Input: part model. Units: mm. Frame: model coordinates. A direction names the side the tool comes from. Coordinates: 2 decimals unless noted, no trailing zeros. Write each loop counter-clockwise with the first axis right and the second up, starting at its lowest first coordinate (ties: lowest second). Pieces come first, ordered by that corner, then holes.
from build123d import *

# Parameters (mm, degrees)
SKETCH1_W           = 81
SKETCH1_H           = 29
BOSS_EXTRUDE1_DEPTH = 3
CUT_EXTRUDE2_DEPTH  = 81
CUT_EXTRUDE3_DEPTH  = 81
SKETCH6_W           = 1.85
SKETCH6_H           = 1.55
CUT_EXTRUDE5_DEPTH  = 0.6
FILLET6_R           = 0.4
CHAMFER2_SIZE       = 0.2
SKETCH7_W           = 1.85
SKETCH7_H           = 1.55
CUT_EXTRUDE6_DEPTH  = 0.6
FILLET7_R           = 0.4
CHAMFER3_SIZE       = 0.2
SKETCH11_W          = 81
SKETCH11_H          = 26.1
CUT_EXTRUDE7_DEPTH  = 0.2
FILLET8_R           = 0.4
BOSS_EXTRUDE2_DEPTH = 3
FILLET9_R           = 1
FILLET10_R          = 0.5


with BuildPart() as part:
    # Sketch1 → Boss-Extrude1 (new body)
    with BuildSketch(Plane(origin=(0, 0, 0), x_dir=(1, 0, 0), z_dir=(0, 1, 0))):
        with Locations((40.5, 14.5)):
            Rectangle(SKETCH1_W, SKETCH1_H)
    extrude(amount=BOSS_EXTRUDE1_DEPTH)

    # Sketch2 → Cut-Extrude2 (cut)
    with BuildSketch(Plane(origin=(81, 0, 0), x_dir=(0, 0, -1), z_dir=(1, 0, 0))):
        Polygon((0, 3), (3, 3), (3, 1.75), (1.25, 1.75), (1.25, 0), (0, 0), align=None)
        Polygon((29, 0), (27.75, 0), (27.75, 1.75), (26, 1.75), (26, 3), (29, 3), align=None)
    extrude(amount=-CUT_EXTRUDE2_DEPTH, mode=Mode.SUBTRACT)

    # Sketch4 → Cut-Extrude3 (cut)
    with BuildSketch(Plane(origin=(81, 0, 0), x_dir=(0, 0, -1), z_dir=(1, 0, 0))):
        Polygon((27.75, 0), (27.55, 0), (27.55, 1.55), (25.8, 1.55), (25.8, 3), (26, 3), (26, 1.75), (27.75, 1.75), align=None)
        Polygon((3.2, 3), (3, 3), (3, 1.75), (1.25, 1.75), (1.25, 0), (1.45, 0), (1.45, 1.55), (3.2, 1.55), align=None)
    extrude(amount=-CUT_EXTRUDE3_DEPTH, mode=Mode.SUBTRACT)

    # Sketch6 → Cut-Extrude5 (cut)
    with BuildSketch(Plane.XY.offset(-1.45)):
        with Locations((3, 0.775)):
            Rectangle(SKETCH6_W, SKETCH6_H)
    extrude(amount=-CUT_EXTRUDE5_DEPTH, mode=Mode.SUBTRACT)

    # Fillet6
    fillet6_edges = [part.edges().sort_by_distance(p)[0] for p in [
        (2.075, 0.775, -1.45),
    ]]
    fillet(fillet6_edges, radius=FILLET6_R)

    # Chamfer2
    chamfer2_edges = [part.edges().sort_by_distance(p)[0] for p in [
        (3.925, 0.775, -1.45),
    ]]
    chamfer(chamfer2_edges, length=CHAMFER2_SIZE)

    # Sketch7 → Cut-Extrude6 (cut)
    with BuildSketch(Plane(origin=(0, 0, -27.55), x_dir=(-1, 0, 0), z_dir=(0, 0, -1))):
        with Locations((-3, 0.775)):
            Rectangle(SKETCH7_W, SKETCH7_H)
    extrude(amount=-CUT_EXTRUDE6_DEPTH, mode=Mode.SUBTRACT)

    # Fillet7
    fillet7_edges = [part.edges().sort_by_distance(p)[0] for p in [
        (2.075, 0.775, -27.55),
    ]]
    fillet(fillet7_edges, radius=FILLET7_R)

    # Chamfer3
    chamfer3_edges = [part.edges().sort_by_distance(p)[0] for p in [
        (3.925, 0.775, -27.55),
    ]]
    chamfer(chamfer3_edges, length=CHAMFER3_SIZE)

    # Sketch11 → Cut-Extrude7 (cut)
    with BuildSketch(Plane(origin=(0, 0, 0), x_dir=(-1, 0, 0), z_dir=(0, -1, 0))):
        with Locations((-40.5, 14.5)):
            Rectangle(SKETCH11_W, SKETCH11_H)
    extrude(amount=-CUT_EXTRUDE7_DEPTH, mode=Mode.SUBTRACT)

    # Fillet8
    fillet8_edges = [part.edges().sort_by_distance(p)[0] for p in [
        (0, 0.875, -27.55),
        (0, 0.875, -1.45),
    ]]
    fillet(fillet8_edges, radius=FILLET8_R)

    # Sketch9 → Boss-Extrude2 (add)
    with BuildSketch(Plane(origin=(0, 3, 0), x_dir=(1, 0, 0), z_dir=(0, 1, 0))):
        with BuildLine():
            Line((74.5, 9.5), (74.5, 19.5))
            ThreePointArc((74.5, 19.5), (76, 21), (77.5, 19.5))
            Line((77.5, 19.5), (77.5, 9.5))
            ThreePointArc((77.5, 9.5), (76, 8), (74.5, 9.5))
        make_face()
    extrude(amount=BOSS_EXTRUDE2_DEPTH)

    # Fillet9
    fillet9_edges = [part.edges().sort_by_distance(p)[0] for p in [
        (76, 6, -8),
        (77.5, 6, -14.5),
        (76, 6, -21),
        (74.5, 6, -14.5),
    ]]
    fillet(fillet9_edges, radius=FILLET9_R)

    # Fillet10
    fillet10_edges = [part.edges().sort_by_distance(p)[0] for p in [
        (76, 3, -8),
        (77.5, 3, -14.5),
        (76, 3, -21),
        (74.5, 3, -14.5),
    ]]
    fillet(fillet10_edges, radius=FILLET10_R)


solid = part.part
Item 1: Pin query (flat end, axial travel): pin 1 Ø1 at (x, y) = (37, 5) entering from -Z; pin 2 Ø0.5 at (x, z) = (31.5, -26.5) entering from +Y; pin 3 Ø3 at (x, y) = (23, 4) entering from -Z; pin 4 Ø1 at (x, z) = (18.5, -5.5) entering from +Y. Return the tip coordinate at first contact, or that it passes through.
Item 2: Section query D-D, the plane z = -24.5. Return loops of the section in (x, y).
Item 3: Section query B-B, the plane z = -13.75. Return loops of the section in (x, y).
Item 4: Material intervals for line 1 (Y direction, x = 28, z = -14.5); line 2 (Y direction, x = 68.5, z = -26.5); line 3 (X direction, y = 4.1, z = -12.5), sorted ascending.
Item 5: Section query A-A, the plane x = 46. Return loops of the section in (y, z), then the cut area to 3 significant figures.
Item 6: Access query for faces 4 (the face through (77.5, 4, -15)), 5 (the face through (41, 2, -25.8)), 6 (the face through (3, 1, -26.95)), 7 (the face through (41, 2, -3.2)). Directions: +Z, -Z, +X, -X, +Y, -Y. A direction counts if a zero-diameter tool reaches every point of the face in a straight line with its end or side. Return the directions, or none.
Item 7: Section query C-C, the plane y = 2.3. Return loops of the section in (x, z), then the cut area to 3 significant figures.
Item 8: Pull-direction query (X, two-part tool) for faces 1 (the face through (3, 1, -2.05)), 2 (the face through (76, 4, -8)), 3 (the face through (43, 1, -27.55)); classes: released by +X, released by -X, zero draft, split by the parting line, or undercut.
The answers:
1. pin 1: passes through
1. pin 2: stops at y = 1.55
1. pin 3: stops at z = -25.8
1. pin 4: stops at y = 3
2. outline: (0, 0.2) - (81, 0.2) - (81, 3) - (0, 3) - close
3. outline: (0, 0.2) - (81, 0.2) - (81, 3) - (78, 3) arc R0.5 cw to (77.5, 3.5) - (77.5, 5) arc R1 ccw to (76.5, 6) - (75.5, 6) arc R1 ccw to (74.5, 5) - (74.5, 3.5) arc R0.5 cw to (74, 3) - (0, 3) - close
4. line 1: y = 0.2 to 3
4. line 2: y = 0.2 to 1.55
4. line 3: x = 74.5 to 77.5
5. outline: (0.2, -27.55) - (1.55, -27.55) - (1.55, -25.8) - (3, -25.8) - (3, -3.2) - (1.55, -3.2) - (1.55, -1.45) - (0.2, -1.45) - close
5. area: 68.0 mm2
6. face 4: +Z, -Z, +X, +Y
6. face 5: -Z, +X, -X, +Y
6. face 6: -Z, +Y, -Y
6. face 7: +Z, +X, -X, +Y
7. outline: (0, -25.8) - (81, -25.8) - (81, -3.2) - (0, -3.2) - close
7. area: 1,830 mm2
8. face 1: undercut
8. face 2: split by the parting line
8. face 3: zero draft
